Model file for the job. Use its own axes, mm. Give positions to 0.01 mm unless a question says otherwise; leave off trailing zeros. Write each loop counter-clockwise with the first axis right and the second up, starting at its lowest first coordinate (ties: lowest second). Pieces come first, ordered by that corner, then holes. Notation, with made-up numbers: (-33, 3) - (26, 3) arc R20 cw to (26, 18) - close; hole circle Ø7 at (-12.5, 69.5). An arc over 180 degrees is marked (long way). One line per item, written item: value. Start each with the question number.
(1) Cut at C-C, the plane z = 10. List the corners of the cut face in (x, y), and give its area (3 significant figures).
(2) Cut at A-A, the plane y = 0. State how many separate pieces and enclosed holes the cut face has, and give its area (3 significant figures).
(3) Cut at B-B, the plane x = 2.5. List the corners of the cut face in (y, z), and give its area (3 significant figures).
(4) Probe L1, parallel to Z at x = -9.3, y = 0; L2, parallel to X at y = -7.75, z = 244; L3, parallel to Y at x = -9.45, z = 490. List the from-to ranges inside material, lowest first.
(5) Drop a flat-ended pin along its axis: P1, Ø2, axis at x = 3, y = 6, coming from the -Z side. Give the stop position or say it passes through.
(6) Cut at D-D, the plane z = 186. List the corners of the cut face in (x, y), and give its area (3 significant figures).
from build123d import *

# Parameters (mm, degrees)
SKETCH1_W           = 20
SKETCH1_H           = 20
SKETCH1_W_2         = 17.6
SKETCH1_H_2         = 17.6
BOSS_EXTRUDE1_DEPTH = 500
SKETCH2_R           = 4.25
CUT_EXTRUDE1_DEPTH  = 600


with BuildPart() as part:
    # Sketch1 → Boss-Extrude1 (new body)
    with BuildSketch(Plane.XY):
        Rectangle(SKETCH1_W, SKETCH1_H)
        Rectangle(SKETCH1_W_2, SKETCH1_H_2, mode=Mode.SUBTRACT)
    extrude(amount=BOSS_EXTRUDE1_DEPTH)

    # Sketch2 → Cut-Extrude1 (cut)
    with BuildSketch(Plane(origin=(10, 0, 0), x_dir=(0, 0, -1), z_dir=(1, 0, 0))):
        with Locations(Location((-490, 0, 0), (0, 0, 90))):
            Circle(SKETCH2_R)
        with Locations(Location((-10, 0, 0), (0, 0, 90))):
            Circle(SKETCH2_R)
        with Locations(Location((-40, 0, 0), (0, 0, 90))):
            Circle(SKETCH2_R)
    extrude(amount=-CUT_EXTRUDE1_DEPTH, mode=Mode.SUBTRACT)


solid = part.part
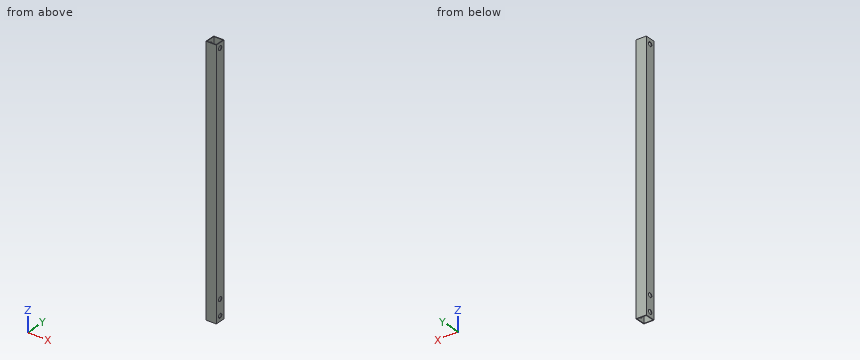
Answers follow:
1. outline: (-10, -10) - (10, -10) - (10, -4.25) - (8.8, -4.25) - (8.8, -8.8) - (-8.8, -8.8) - (-8.8, -4.25) - (-10, -4.25) - close; (-10, 4.25) - (-8.8, 4.25) - (-8.8, 8.8) - (8.8, 8.8) - (8.8, 4.25) - (10, 4.25) - (10, 10) - (-10, 10) - close
1. area: 69.8 mm²
2. separate pieces: 8
2. enclosed holes: 0
2. area: 1,140 mm²
3. outline: (-10, 0) - (-8.8, 0) - (-8.8, 500) - (-10, 500) - close; (8.8, 0) - (10, 0) - (10, 500) - (8.8, 500) - close
3. area: 1,200 mm²
4. L1: z = 0 to 5.75, 14.25 to 35.75, 44.25 to 485.75, 494.25 to 500
4. L2: x = -10 to -8.8, 8.8 to 10
4. L3: y = -10 to -4.25, 4.25 to 10
5. P1: passes through
6. outline: (-10, -10) - (10, -10) - (10, 10) - (-10, 10) - close; hole (-8.8, -8.8) - (8.8, -8.8) - (8.8, 8.8) - (-8.8, 8.8) - close
6. area: 90.2 mm²
